Here's how the part is built. I have some questions about the finished solid (model axes, mm). Round coordinates to 2 decimals unless told otherwise and drop trailing zeros. Write each loop counter-clockwise with the first axis right and the second up, starting at its lowest first coordinate (ties: lowest second). Pieces come first, ordered by that corner, then holes. Notation, with made-up numbers: (3.5, -5) -> (21.5, -5) arc R31 cw to (21.5, 28) -> close; hole circle Ø6 at (71, 52.5). An arc over 180 degrees is marked (long way). Answer as CSV lines item,"result".
Autodesk Inventor part; units mm, degrees
ref_plane "YZ Plane" through (0, 0, 0) normal (1, 0, 0) x (0, 1, 0)
ref_plane "XZ Plane" through (0, 0, 0) normal (0, 1, 0) x (-1, 0, 0)
ref_plane "XY Plane" through (0, 0, 0) normal (0, 0, 1) x (1, 0, 0)
sketch "Sketch2" plane through (0, 0, 0) normal (1, 0, 0) x (0, 1, 0)
  line L0 (63.5, 38.1) -> (-63.5, 38.1) construction
  line L1 (-63.5, 38.1) -> (-63.5, -38.1) construction
  line L2 (-63.5, -38.1) -> (63.5, -38.1) construction
  line L3 (63.5, -38.1) -> (63.5, 38.1) construction
  line L4 (63.5, 38.1) -> (-63.5, -38.1) construction
  line L5 (-63.5, 38.1) -> (63.5, -38.1) construction
  line L6 (-63.5, 38.1) -> (-76.2, 38.1) construction
  line L7 (-76.2, 38.1) -> (-76.2, -266.7) construction
  line L8 (-76.2, -266.7) -> (-63.5, -266.7) construction
  line L9 (-63.5, -266.7) -> (-63.5, 38.1) construction
  circle A0 centre (-25.8145, -515.3533) radius 57.15 construction
  circle A1 centre (-50.8, -140.0055) radius 15.875 construction
  circle A2 centre (19.05, -69.85) radius 25.4 construction
  circle A3 centre (98.425, -260.3407) radius 63.5 construction
  circle A4 centre (98.425, -260.3407) radius 14.1605
  circle A5 centre (172.9213, -164.3575) radius 63.5 construction
  circle A6 centre (172.9213, -164.3575) radius 14.1605
  circle A7 centre (-50.8, -140.0055) radius 14.1605
  circle A8 centre (19.05, -69.85) radius 14.1605
  line L10 (-69.85, 38.1) -> (-69.85, -155.1245)
  line L11 (-57.15, 38.1) -> (-6.35, 38.1) construction
  line L12 (-6.35, 38.1) -> (-6.35, 444.5) construction
  line L13 (-6.35, 444.5) -> (-57.15, 444.5) construction
  line L14 (-57.15, 444.5) -> (-57.15, 38.1) construction
  line L15 (172.9213, -185.376) -> (172.9213, -143.339) construction
  line L16 (98.425, -239.3222) -> (98.425, -281.3592) construction
  line L17 (19.05, -48.8315) -> (19.05, -90.8685) construction
  line L18 (-50.8, -118.987) -> (-50.8, -161.024) construction
  circle A9 centre (98.425, -281.3592) radius 6.35 construction
  circle A10 centre (98.425, -260.3407) radius 20.5105 construction
  circle A11 centre (172.9213, -164.3575) radius 20.5105 construction
  circle A12 centre (-50.8, -140.0055) radius 24.3205 construction
  line L19 (234.95, -119.0025) -> (103.4052, -285.2987)
  line L20 (-65.9175, -159.0567) -> (94.4779, -286.3334)
  arc A13 (-69.85, -124.8864) -> (-65.9175, -159.0567) centre (-50.8, -140.0055) ccw
  arc A14 (94.4779, -286.3334) -> (103.4052, -285.2987) centre (98.425, -281.3592) ccw
  line L21 (-69.85, 38.1) -> (-69.85, 190.5)
  line L22 (-69.85, 190.5) -> (234.95, 190.5)
  line L23 (234.95, 190.5) -> (234.95, -119.0025)
  line L24 (199.0311, -58.2205) -> (108.7364, 11.8607)
  line L25 (108.7364, 11.8607) -> (-76.2, -226.4168)
  line L26 (-76.2, -226.4168) -> (14.0946, -296.4979)
  line L27 (14.0946, -296.4979) -> (199.0311, -58.2205)
  circle A15 centre (172.9213, -164.3575) radius 44.45 construction
  circle A16 centre (98.425, -260.3407) radius 44.45 construction
  line L28 (63.5, 38.1) -> (63.5, 190.5) construction
  line L29 (152.4, 38.1) -> (152.4, 190.5) construction
  line L30 (222.25, 114.3) -> (82.55, 114.3) construction
  point P0 (0, 0)
  point P1 (-14.3002, 165.1)
  point P2 (-49.1998, 165.1)
  point P3 (-14.3002, 190.5)
  point P4 (-49.1998, 190.5)
  point P5 (-14.3002, 215.9)
  point P6 (-49.1998, 215.9)
  point P7 (-14.3002, 241.3)
  point P8 (-49.1998, 241.3)
  point P9 (-31.75, 38.1)
  point P10 (222.25, 177.8)
  point P11 (222.25, 165.1)
  point P12 (222.25, 152.4)
  point P13 (222.25, 139.7)
  point P14 (222.25, 127)
  point P15 (222.25, 101.6)
  point P16 (222.25, 88.9)
  point P17 (222.25, 76.2)
  point P18 (222.25, 63.5)
  point P19 (222.25, 50.8)
  point P20 (222.25, 38.1)
  point P21 (63.5, 114.3)
  point P22 (152.4, 114.3)
  point P23 (152.4, 114.3)
  point P24 (152.4, 114.3)
  point P25 (82.55, 177.8)
  point P26 (82.55, 165.1)
  point P27 (82.55, 152.4)
  point P28 (82.55, 139.7)
  point P29 (82.55, 127)
  point P30 (82.55, 101.6)
  point P31 (82.55, 88.9)
  point P32 (82.55, 76.2)
  point P33 (82.55, 63.5)
  point P34 (82.55, 50.8)
  point P35 (82.55, 38.1)
  dimension "d2" = 127
  dimension "d3" = 76.2
  dimension "d4" = 12.7
  dimension "d5" = 304.8
  dimension "d6" = 114.3
  dimension "d7" = 31.75
  dimension "d8" = 50.8
  dimension "d9" = 127
  dimension "d10" = 174.625
  dimension "d11" = 28.321
  dimension "d12" = 31.75
  dimension "d13" = 25.4
  dimension "d14" = 98.999
  dimension "d16" = 222.2407
  dimension "d17" = 127
  dimension "d18" = 121.5009
  dimension "d40" = 50.8
  dimension "d41" = 19.05
  dimension "d42" = 406.4
  dimension "d43" = 127
  dimension "d44" = 7.9502
  dimension "d45" = 7.9502
  dimension "d48" = 25.4
  dimension "d70" = 180.577
  dimension "d80" = 42.037
  dimension "d81" = 42.037
  dimension "d82" = 42.037
  dimension "d83" = 42.037
  dimension "d84" = 12.7
  dimension "d85" = 6.35
  dimension "d86" = 6.35
  dimension "d87" = 10.16
  dimension "d97" = 152.4
  dimension "d98" = 12.7
  dimension "d101" = 12.7
  dimension "d104" = 12.7
  dimension "d109" = 114.3
  dimension "d110" = 301.625
  dimension "d111" = 19.05
  dimension "d112" = 95.25
  dimension "d113" = 304.8
  dimension "d114" = 139.7
extrude "Extrusion1" add sketch "Sketch2" along normal blind 6.35 contours L21 L22 L23 L19 A14 L20 L27 L24 L25 A13 L10 | L10 A13 | L25 L24 L27 L20
sketch "Sketch3" plane through (6.35, 0, 0) normal (1, 0, 0) x (0, 0, -1)
  line L0 (-38.1, 63.5) -> (38.1, 63.5) construction
  line L1 (38.1, 63.5) -> (38.1, -63.5) construction
  line L2 (38.1, -63.5) -> (-38.1, -63.5) construction
  line L3 (-38.1, -63.5) -> (-38.1, 63.5) construction
  line L4 (-38.1, 63.5) -> (38.1, -63.5) construction
  line L5 (38.1, 63.5) -> (-38.1, -63.5) construction
  line L6 (-190.5, -69.85) -> (124.8864, -69.85) construction
  point P0 (0, 0)
  point P1 (0, 0)
  point P2 (147.943, -69.85)
  dimension "d36" = 76.2
  dimension "d37" = 127
  dimension "d38" = 6.35
sketch "Sketch4" plane through (0, 0, 0) normal (-1, 0, 0) x (0, 0, 1)
  circle A0 centre (-5.796, 31.75) radius 10.16
  line L0 (190.5, -69.85) -> (-124.8864, -69.85)
  line L1 (190.5, -69.85) -> (-124.8864, -69.85)
  circle A1 centre (-5.796, 31.75) radius 25.4 construction
  circle A2 centre (-69.85, 19.05) radius 14.1605
  circle A3 centre (-140.0055, -50.8) radius 14.1605
  circle A4 centre (-164.3575, 172.9213) radius 14.1605
  circle A5 centre (-260.3407, 98.425) radius 14.1605
  arc A6 (-159.0567, -65.9175) -> (-124.8864, -69.85) centre (-140.0055, -50.8) ccw
  line L2 (-159.0567, -65.9175) -> (-286.3334, 94.4779)
  arc A7 (-285.2987, 103.4052) -> (-286.3334, 94.4779) centre (-281.3592, 98.425) ccw
  line L3 (-285.2987, 103.4052) -> (-119.0025, 234.95)
  line L4 (-119.0025, 234.95) -> (190.5, 234.95)
  line L5 (190.5, 234.95) -> (190.5, -69.85)
  circle A8 centre (-69.85, 19.05) radius 14.1605
  circle A9 centre (-140.0055, -50.8) radius 14.1605
  circle A10 centre (-164.3575, 172.9213) radius 14.1605
  circle A11 centre (-260.3407, 98.425) radius 14.1605
  arc A12 (-159.0567, -65.9175) -> (-124.8864, -69.85) centre (-140.0055, -50.8) ccw
  line L6 (-159.0567, -65.9175) -> (-286.3334, 94.4779)
  arc A13 (-285.2987, 103.4052) -> (-286.3334, 94.4779) centre (-281.3592, 98.425) ccw
  line L7 (-285.2987, 103.4052) -> (-119.0025, 234.95)
  line L8 (-119.0025, 234.95) -> (190.5, 234.95)
  line L9 (190.5, 234.95) -> (190.5, -69.85)
  point P0 (0, 0)
  point P1 (-69.85, -12.7)
  point P2 (-5.796, 57.15)
  point P3 (-27.7931, 44.45)
  point P4 (-27.7931, 19.05)
  point P5 (-5.796, 6.35)
  point P6 (16.201, 19.05)
  point P7 (16.201, 44.45)
  dimension "d58" = 50.8
  dimension "d53" = 20.32
  dimension "d55" = 101.6
  dimension "d61" = 360
  dimension "d117" = 65.3009
extrude "Extrusion2" cut sketch "Sketch4" against normal blind 25.4 contours A0
hole "Hole1" at (0, 57.15, -5.796) at (0, 44.45, -27.7931) at (0, 19.05, -27.7931) at (0, 6.35, -5.796) at (0, 19.05, 16.201) at (0, 44.45, 16.201) direction (1, 0, 0) diameter 5.1054 end through all
hole "Hole3" at (0, -14.3002, 215.9) at (0, -49.1998, 215.9) at (0, -14.3002, 241.3) at (0, -49.1998, 241.3) at (0, 172.9213, -185.376) at (0, 172.9213, -143.339) at (0, 98.425, -239.3222) at (0, 98.425, -281.3592) at (0, 19.05, -48.8315) at (0, 19.05, -90.8685) at (0, -50.8, -118.987) at (0, -50.8, -161.024) at (0, 222.25, 177.8) at (0, 222.25, 165.1) at (0, 222.25, 152.4) at (0, 222.25, 139.7) at (0, 222.25, 127) at (0, 222.25, 114.3) at (0, 222.25, 101.6) at (0, 222.25, 88.9) at (0, 222.25, 76.2) at (0, 222.25, 63.5) at (0, 222.25, 50.8) at (0, 222.25, 38.1) at (0, 82.55, 38.1) at (0, 82.55, 50.8) at (0, 82.55, 63.5) at (0, 82.55, 76.2) at (0, 82.55, 88.9) at (0, 82.55, 101.6) at (0, 82.55, 114.3) at (0, 82.55, 127) at (0, 82.55, 139.7) at (0, 82.55, 152.4) at (0, 82.55, 165.1) at (0, 82.55, 177.8) direction (1, 0, 0) diameter 5.1054 end through all
sketch "Sketch6" plane through (6.35, 0, 0) normal (1, 0, 0) x (0, 0, -1)
  line L0 (-190.5, -69.85) -> (124.8864, -69.85)
  line L1 (-190.5, -69.85) -> (-38.1, -69.85)
  line L2 (-38.1, -69.85) -> (-38.1, 57.15)
  line L3 (-38.1, 57.15) -> (-190.5, 57.15)
  line L4 (-190.5, 57.15) -> (-190.5, -69.85)
  point P0 (0, 0)
  dimension "d115" = 127
  dimension "d116" = 152.4
properties part number "GI - 001" material "Aluminum 6061"
Item 1: Will this pin go through, and if not, where does the flat tip stop? pin 1 (1 mm diameter, centred on x = 3.5, z = 95, fed in from -Y).
Results found:
pin 1,"stops at y = -69.85"
Item 2: If we mould it in two halves opening along Y, with no side actions, what happens to faces 1 (the flat face through (3.131, 170.098, -200.987)), 2 (the cylindrical face through (3.13, 21.83, -8)), 3 (the flat face through (6.35, 78, 8)), 4 (the flat face through (3.131, 13.157, -221.804))? For each: pulls with the +Y half, pulls with the -Y half, needs draft (parallel to the pull), parting line crosses it, or undercut.
Results found:
face 1,"pulls with the +Y half"
face 2,"undercut"
face 3,"needs draft"
face 4,"pulls with the -Y half"
Item 3: Suppose I cut it at B-B, the plane x = 4.5. State how many separate pieces and enclosed holes the cut face has, then the cut area to 3 significant figures.
Results found:
separate pieces,"1"
enclosed holes,"43"
area,"120,000 mm²"
Item 4: Suppose I cut it at A-A, the plane z = -69.85. List the corners of the cut face in (x, y) for me.
Results found:
outline,"(0, -69.85) -> (6.35, -69.85) -> (6.35, 4.89) -> (0, 4.89) -> close; (0, 33.21) -> (6.35, 33.21) -> (6.35, 234.95) -> (0, 234.95) -> close"
Item 5: I need wall thicknesses on L1, parallel to Y at x = 2.75, z = 50.8; L2, parallel to Z at x = 3.5, y = 24; L3, parallel to Y at x = 1.5, z = 21.5. Which ranges of each line are inside material? Lowest first, please.
Results found:
L1,"y = -69.85 to 80, 85.1 to 219.7, 224.8 to 234.95"
L2,"z = -230.41 to -83.12, -56.58 to -12.37, 0.77 to 190.5"
L3,"y = -69.85 to 234.95"
Item 6: Suppose I cut it at C-C, the plane y = 203. List the corners of the cut face in (x, z) for me, then the cut area to 3 significant figures.
Results found:
outline,"(0, -159.39) -> (6.35, -159.39) -> (6.35, 190.5) -> (0, 190.5) -> close"
area,"2,220 mm²"
